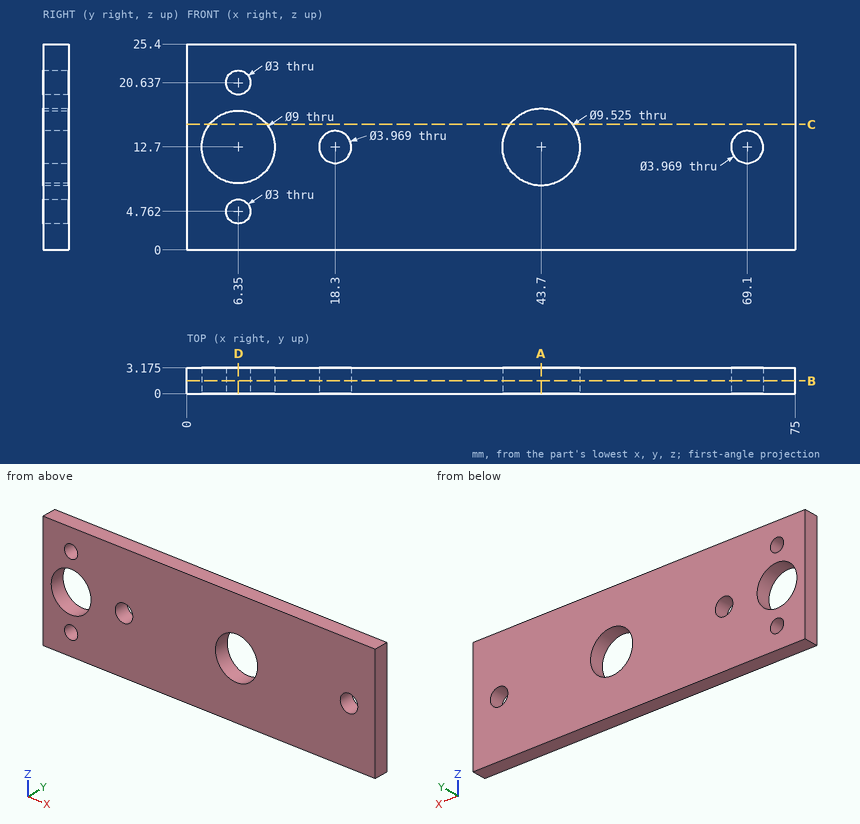
Geometry check sheet. Reference: drawing and pictorial views, mm from the part's lowest x, y, z. Round coordinates to 2 decimals unless told otherwise and drop trailing zeros. Order: outer loops, then holes, each group sorted by start corner. A loop starts at its lowest first (then second) coordinate and runs counter-clockwise, first axis right, second up. Notation, with made-up numbers: (-13, -29) -> (5, -29) arc R10 ccw to (5, -17) -> close; hole circle Ø7 at (41, 42.25). An arc over 180 degrees is marked (long way). One line per item, written item: value. Start each with the question number.
Q1. Cross-section at B-B (y = 1.6). Give the number of separate pieces and of enclosed holes in the cut face, and give its area (3 significant figures).
Q2. Gauge pin test, flat ends, axial feed: pin 1 Ø14.5 at (x, z) = (6.35, 12.7) entering from +Y (1 decimal); pin 2 Ø3 at (x, z) = (69.1, 12.7) entering from +Y. Record the tip position at first contact, or that the pin passes through.
Q3. Cross-section at A-A (x = 43.7). Record the boundary of the cut face in (y, z) (1 decimal).
Q4. Cross-section at D-D (x = 6.35). Record the boundary of the cut face in (y, z) (1 decimal).
Q5. Thickness scan on line 1 (Z direction, x = 46, y = 1.35); line 2 (X direction, y = 2.35, z = 13.5) (1 decimal); line 3 (Z direction, x = 9, y = 1.15) (1 decimal). Record the ranges inside material, lowest first.
Q6. Cross-section at C-C (z = 15.5). Record the boundary of the cut face in (x, y) (1 decimal), and give its area (3 significant figures).
Completed:
1. separate pieces: 1
1. enclosed holes: 6
1. area: 1,730 mm²
2. pin 1: stops at y = 3.2
2. pin 2: passes through
3. outline: (0, 0) -> (3.2, 0) -> (3.2, 7.9) -> (0, 7.9) -> close; (0, 17.5) -> (3.2, 17.5) -> (3.2, 25.4) -> (0, 25.4) -> close
4. outline: (0, 0) -> (3.2, 0) -> (3.2, 3.3) -> (0, 3.3) -> close; (0, 6.3) -> (3.2, 6.3) -> (3.2, 8.2) -> (0, 8.2) -> close; (0, 17.2) -> (3.2, 17.2) -> (3.2, 19.1) -> (0, 19.1) -> close; (0, 22.1) -> (3.2, 22.1) -> (3.2, 25.4) -> (0, 25.4) -> close
5. line 1: z = 0 to 8.53, 16.87 to 25.4
5. line 2: x = 0 to 1.9, 10.8 to 16.5, 20.1 to 39, 48.4 to 67.3, 70.9 to 75
5. line 3: z = 0 to 9.1, 16.3 to 25.4
6. outline: (0, 0) -> (2.8, 0) -> (2.8, 3.2) -> (0, 3.2) -> close; (9.9, 0) -> (39.8, 0) -> (39.8, 3.2) -> (9.9, 3.2) -> close; (47.6, 0) -> (75, 0) -> (75, 3.2) -> (47.6, 3.2) -> close
6. area: 191 mm²
